Check sheet for the modelled part. Datum: model origin and axes. Units: mm. A direction names the side the tool comes from. Round coordinates to 2 decimals unless told otherwise and drop trailing zeros. Loops run counter-clockwise (first coordinate to the right, second up) from the corner with the lowest first, then second, coordinate; pieces in that order, holes last. Notation, with made-up numbers: M -18.5,-26.75 L 1.5,-26.75 A11 ccw 1.5,-13.75 Z; hole C -24,50.25 d7. An arc over 180 degrees is marked long. Write item = value, one per line. Start each with the question number.
(1) Mould release check, pull along X, two halves, no side actions. Record for faces 6 (the face through (-6, -11, 0)), 7 (the face through (78, -8, 0)), 8 (the face through (42.11, -3.45, 0.1)): pulls with the +X half, pulls with the -X half, needs draft (parallel to the pull), parting line crosses it, or undercut.
(2) Set-up check for faces 1 (the face through (9, -7, 0)), 2 (the face through (44, -7, -7)), 3 (the face through (45, -7, 7)), 4 (the face through (78, 0, 0)), 5 (the face through (-12.49, -10.94, 0.45)): record each of +Z, -Z, +X, -X, +Y, -Y from which the full face is reachable in a straight line by a thin tool's end or side.
(3) Scan lines: L1, parallel to Z at x = 0, y = -12.75; L2, parallel to Z at x = 85, y = -1.5; L3, parallel to Z at x = 33, y = -7.25. Record each from-to range of solid material in increasing order. Write a range as from..to.
(4) Cross-section at D-D on y = -2.25. Record the boundary of the cut face in (x, z), plus the area to 3 significant figures.
(5) Cross-section at B-B on y = -12.75. Record the boundary of the cut face in (x, z).
(6) Cross-section at C-C on x = 0. Record the boundary of the cut face in (y, z), plus the area to 3 significant figures.
(7) Cross-section at A-A on x = 85. Record the boundary of the cut face in (y, z).
(8) Go/stop test with flat-tipped pins: P1, Ø1, axis at x = 39.5, z = 4.5, coming from the -Y side; P2, Ø3, axis at y = -9, z = -3, coming from the -X side; P3, Ø4, axis at x = 51.5, z = 5, coming from the -Y side; P4, Ø1.5, axis at x = 21.5, y = -5.5, coming from the +Z side. Record where each tip stops, or that it passes through.
from build123d import *

# Parameters (mm, degrees)
F0_R     = 6
F1_DEPTH = 20
F3_DEPTH = 12.5


with BuildPart() as f1:
    # F0 (on Front) → F1 (new body)
    with BuildSketch(Plane.XZ):
        with BuildLine():
            ThreePointArc((10.356158, -7), (11.952028, -3.660467), (12.5, 0))
            ThreePointArc((12.5, 0), (11.952028, 3.660467), (10.356158, 7))
            ThreePointArc((10.356158, 7), (-12.5, 0), (10.356158, -7))
        make_face()
        Circle(F0_R, mode=Mode.SUBTRACT)
        with BuildLine():
            ThreePointArc((10.356158, 7), (11.952028, 3.660467), (12.5, 0))
            ThreePointArc((12.5, 0), (11.952028, -3.660467), (10.356158, -7))
            Line((10.356158, -7), (77.858572, -7))
            ThreePointArc((77.858572, -7), (75, 0), (77.858572, 7))
            Line((77.858572, 7), (10.356158, 7))
        make_face()
        with BuildLine():
            ThreePointArc((95, 0), (88.78059, 9.257815), (77.858572, 7))
            ThreePointArc((77.858572, 7), (75, 0), (77.858572, -7))
            ThreePointArc((77.858572, -7), (88.78059, -9.257815), (95, 0))
        make_face()
        with Locations((85, 0)):
            Circle(F0_R, mode=Mode.SUBTRACT)
    extrude(amount=F1_DEPTH)

    # F2 (on Top) → F3 (intersect, symmetric)
    with BuildSketch(Plane.XY):
        Polygon((95, -8), (95, 0), (81.679874, 0), (61.679874, 0), (21.980901, -7), (-12.5, -7), (-12.5, -15), (22.68081, -15), (62.379783, -8), (85.50881, -8), align=None)
    extrude(amount=F3_DEPTH, both=True, mode=Mode.INTERSECT)


solid = f1.part
Result:
q1.face_6 = undercut
q1.face_7 = needs draft
q1.face_8 = pulls with the -X half
q2.face_1 = +Z, -Z, -X, +Y
q2.face_2 = -Z, +Y, -Y
q2.face_3 = +Z, +Y, -Y
q2.face_4 = +Z, -Z, +X, -X, +Y
q2.face_5 = +Y, -Y
q3.L1 = -12.5..-6, 6..12.5
q3.L2 = -10..-6, 6..10
q3.L3 = -7..7
q4.outline = M 48.92,-7 L 77.86,-7 A10 ccw long 77.86,7 L 48.92,7 Z; hole C 85,0 d12
q4.area = 579 mm^2
q5.outline = M 10.36,-7 L 35.44,-7 L 35.44,7 L 10.36,7 A12.5 ccw long Z; hole C 0,0 d12
q6.outline = M -15,-12.5 L -7,-12.5 L -7,-6 L -15,-6 Z; M -15,6 L -7,6 L -7,12.5 L -15,12.5 Z
q6.area = 104 mm^2
q7.outline = M -8,-10 L 0,-10 L 0,-6 L -8,-6 Z; M -8,6 L 0,6 L 0,10 L -8,10 Z
q8.P1 = -12.12
q8.P2 = -12.41
q8.P3 = -10.27
q8.P4 = through
